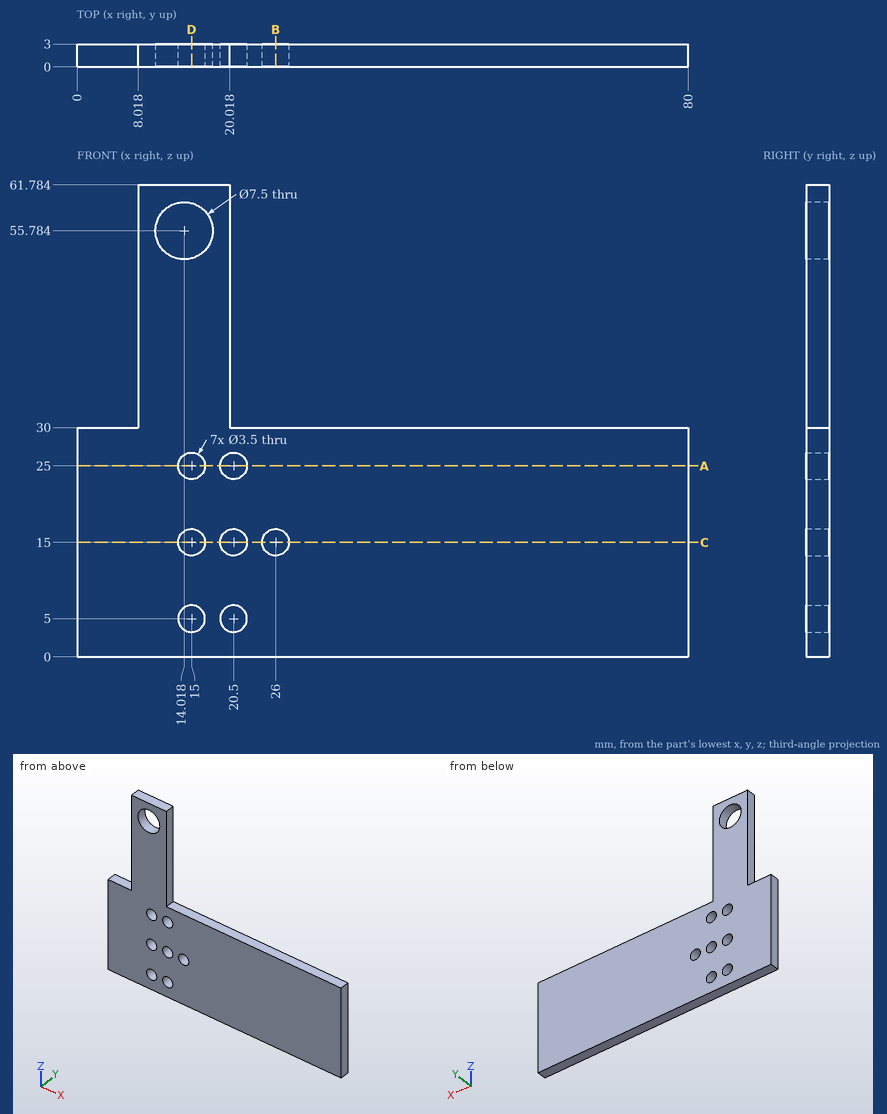
Geometry check sheet. Reference: drawing and pictorial views, mm from the part's lowest x, y, z. Round coordinates to 2 decimals unless told otherwise and drop trailing zeros. Loops run counter-clockwise (first coordinate to the right, second up) from the corner with the lowest first, then second, coordinate; pieces in that order, holes last. Notation, with made-up numbers: M 43.25,-2.75 L 57.25,-2.75 A31 ccw 57.25,36.25 Z; hole C 80,-21 d3. An arc over 180 degrees is marked long. Return JSON: item names as keys, results as strings. Group by question number.
(1) Section check B-B, the plane x = 26. Enter the section's corners in (y, z).
(2) Section check A-A, the plane z = 25. Enter the section's corners in (x, y), and give its area (3 significant figures).
(3) Section check D-D, the plane x = 15. Give the number of separate pieces and of enclosed holes in the cut face, and give its area (3 significant figures).
(4) Scan lines: line 1 along X through (y, z) = (0.85, 25); line 2 along X through (y, z) = (0.95, 15); line 3 along Z through (x, y) = (16.5, 2.45) (1 decimal). Record each from-to range of solid material in increasing order. Write a range as [from, to].
(5) Go/stop test with flat-tipped pins: pin 1 (4 mm diameter, centred on x = 20.5, z = 15, fed in from +Y); pin 2 (1 mm diameter, centred on y = 2.5, z = 32, fed in from -X); pin 3 (0.9 mm diameter, centred on x = 5, y = 1.5, fed in from +Z). Record where each tip stops, or that it passes through.
(6) Section check C-C, the plane z = 15. Enter the section's corners in (x, y).
Data:
{
 "1": {"outline": "M 0,0 L 3,0 L 3,13.25 L 0,13.25 Z; M 0,16.75 L 3,16.75 L 3,30 L 0,30 Z"},
 "2": {"outline": "M 0,0 L 13.25,0 L 13.25,3 L 0,3 Z; M 16.75,0 L 18.75,0 L 18.75,3 L 16.75,3 Z; M 22.25,0 L 80,0 L 80,3 L 22.25,3 Z", "area": "219 mm²"},
 "3": {"separate pieces": "5", "enclosed holes": "0", "area": "132 mm²"},
 "4": {"line 1": "[0, 13.25], [16.75, 18.75], [22.25, 80]", "line 2": "[0, 13.25], [16.75, 18.75], [22.25, 24.25], [27.75, 80]", "line 3": "[0, 4.1], [5.9, 14.1], [15.9, 24.1], [25.9, 53], [58.6, 61.8]"},
 "5": {"pin 1": "y = 3", "pin 2": "x = 8.02", "pin 3": "z = 30"},
 "6": {"outline": "M 0,0 L 13.25,0 L 13.25,3 L 0,3 Z; M 16.75,0 L 18.75,0 L 18.75,3 L 16.75,3 Z; M 22.25,0 L 24.25,0 L 24.25,3 L 22.25,3 Z; M 27.75,0 L 80,0 L 80,3 L 27.75,3 Z"}
}
